Here's how the part is built. I have some questions about the finished solid (model axes, mm). A direction names the side the tool comes from. Coordinates: 2 decimals unless noted, no trailing zeros. Loops run counter-clockwise (first coordinate to the right, second up) from the corner with the lowest first, then second, coordinate; pieces in that order, holes last. Notation, with made-up numbers: M 15,13 L 19,13 A8 cw 19,18 Z; hole C 46,88 d2. An arc over 180 degrees is marked long. Use one line per item in the form item = value. Start each with the question number.
(1) Please list where these lines run through material, in increasing order: L1, parallel to X at y = -1.5, z = 1.5; L2, parallel to Z at x = 45.5, y = -1.3; L3, parallel to Z at x = 42, y = -1.
(2) Imagine slicing it at C-C, the plane z = 81. Please give me the cut outline in (x, y), and give its area (3 significant figures).
(3) On a 3-axis mill with a long thin cutter (end or side, diameter ignored), from which of +Z, -Z, +X, -X, +Y, -Y can I reach the whole of each face in a straight line? I mean faces 5 (the flat face through (14.527, -1.503, 40.216)), 6 (the flat face through (3, -3.048, 42)). Say none if no direction works.
(4) Thinking about a two-plate mould opening in Z: for faces 1 (the flat face through (-14.004, -1.503, 31.367)), 2 (the flat face through (3, 0, 42)), 3 (the flat face through (12.494, -1.503, 90.191)), 4 (the cylindrical face through (15.18, -1.5, 12.8)), which applies, +Z half, -Z half, draft (parallel to the pull), parting line (faces both ways), or undercut?
(5) Will this pin go through, and if not, where does the flat tip stop? P1, Ø1, axis at y = -0.5, z = 55.5, coming from the -X side.
(6) Imagine slicing it at B-B, the plane x = 6. Please give me the cut outline in (y, z).
(7) Imagine slicing it at A-A, the plane y = -1.85. State how many separate pieces and enclosed holes the cut face has, and give its area (3 significant figures).
```python
from build123d import *

# Parameters (mm, degrees)
F0_R     = 3.175
F1_DEPTH = 3.048


with BuildPart() as f1:
    # F0 (on Front) → F1 (new body)
    with BuildSketch(Plane.XZ):
        with BuildLine():
            Line((12.1285329959, 0), (3.175, 0))
            ThreePointArc((3.175, 0), (-2.2450640303, -2.2450640303), (0, 3.175))
            Line((0, 3.175), (0, 12.1285329959))
            ThreePointArc((0, 12.1285329959), (-8.8255371973, 8.3193272451), (-12.1074052539, -0.7155771445))
            ThreePointArc((-12.1074052539, -0.7155771445), (-7.858618829, -9.2381503956), (1.2349249899, -12.0654992811))
            ThreePointArc((1.2349249899, -12.0654992811), (9.002198096, -8.1278374782), (12.1285329959, 0))
        make_face()
        with BuildLine():
            ThreePointArc((0, 12.1285329959), (8.5761679272, 8.5761679272), (12.1285329959, 0))
            Line((12.1285329959, 0), (36.8473577956, 0))
            ThreePointArc((36.8473577956, 0), (39.3551513268, 5.6429323481), (45.2240996253, 7.5631301892))
            Line((45.2240996253, 7.5631301892), (20.3690705941, 10.1070859559))
            ThreePointArc((20.3690705941, 10.1070859559), (15.1229915635, 12.8646775774), (13.2422076318, 18.4850253022))
            Line((13.2422076318, 18.4850253022), (15.8473459627, 62.563383249))
            ThreePointArc((15.8473459627, 62.563383249), (10.8891421627, 51.9482811685), (0, 47.625))
            Line((0, 47.625), (0, 12.1285329959))
        make_face()
        with BuildLine():
            Line((36.8473577956, 0), (12.1285329959, 0))
            ThreePointArc((12.1285329959, 0), (9.002198096, -8.1278374782), (1.2349249899, -12.0654992811))
            Line((1.2349249899, -12.0654992811), (45.2240996253, -7.5631301892))
            ThreePointArc((45.2240996253, -7.5631301892), (39.3551513268, -5.6429323481), (36.8473577956, 0))
        make_face()
        with BuildLine():
            ThreePointArc((-12.1074052539, -0.7155771445), (-8.8255371973, 8.3193272451), (0, 12.1285329959))
            Line((0, 12.1285329959), (0, 47.625))
            ThreePointArc((0, 47.625), (-10.8891421627, 51.9482811685), (-15.8473459627, 62.563383249))
            Line((-15.8473459627, 62.563383249), (-12.1074052539, -0.7155771445))
        make_face()
        with BuildLine():
            ThreePointArc((45.2240996253, 7.5631301892), (39.3551513268, 5.6429323481), (36.8473577956, 0))
            ThreePointArc((36.8473577956, 0), (39.3551513268, -5.6429323481), (45.2240996253, -7.5631301892))
            ThreePointArc((45.2240996253, -7.5631301892), (50.0929323481, -5.0948486732), (52.0526422044, 0))
            ThreePointArc((52.0526422044, 0), (50.0929323481, 5.0948486732), (45.2240996253, 7.5631301892))
        make_face()
        with BuildLine():
            ThreePointArc((47.625, 0), (44.45, -3.175), (41.275, 0))
            ThreePointArc((41.275, 0), (44.45, 3.175), (47.625, 0))
        make_face(mode=Mode.SUBTRACT)
        with BuildLine():
            ThreePointArc((-15.8473459627, 62.563383249), (-10.8891421627, 51.9482811685), (0, 47.625))
            Line((0, 47.625), (0, 60.325))
            ThreePointArc((0, 60.325), (-3.175, 63.5), (0, 66.675))
            Line((0, 66.675), (0, 79.375))
            ThreePointArc((0, 79.375), (-10.4661659349, 75.4362890222), (-15.7388575186, 65.5746057477))
            ThreePointArc((-15.7388575186, 65.5746057477), (-15.8647069883, 64.071574295), (-15.8473459627, 62.563383249))
        make_face()
        with BuildLine():
            Line((0, 60.325), (0, 47.625))
            ThreePointArc((0, 47.625), (10.8891421627, 51.9482811685), (15.8473459627, 62.563383249))
            ThreePointArc((15.8473459627, 62.563383249), (15.8680849846, 63.0314875444), (15.875, 63.5))
            ThreePointArc((15.875, 63.5), (15.8409278154, 64.5395340042), (15.7388575186, 65.5746057477))
            ThreePointArc((15.7388575186, 65.5746057477), (10.4661659349, 75.4362890222), (0, 79.375))
            Line((0, 79.375), (0, 66.675))
            ThreePointArc((0, 66.675), (2.2450640303, 65.7450640303), (3.175, 63.5))
            ThreePointArc((3.175, 63.5), (2.2450640303, 61.2549359697), (0, 60.325))
        make_face()
        with BuildLine():
            Line((-9.1570523114, 115.5070300106), (-15.7388575186, 65.5746057477))
            ThreePointArc((-15.7388575186, 65.5746057477), (-10.4661659349, 75.4362890222), (0, 79.375))
            Line((0, 79.375), (0, 105.0637383927))
            ThreePointArc((0, 105.0637383927), (-6.9446732617, 108.2106616314), (-9.1570523114, 115.5070300106))
        make_face()
        with Locations((-3.6322516389, 98.6820235848)):
            Circle(F0_R, mode=Mode.SUBTRACT)
        with BuildLine():
            Line((0, 105.0637383927), (0, 79.375))
            ThreePointArc((0, 79.375), (10.4661659349, 75.4362890222), (15.7388575186, 65.5746057477))
            Line((15.7388575186, 65.5746057477), (9.1570523114, 115.5070300106))
            ThreePointArc((9.1570523114, 115.5070300106), (9.2164380099, 114.9048131032), (9.2362616073, 114.3))
            ThreePointArc((9.2362616073, 114.3), (6.5310232154, 107.7689767846), (0, 105.0637383927))
        make_face()
        with BuildLine():
            ThreePointArc((9.1570523114, 115.5070300106), (0, 123.5362616073), (-9.1570523114, 115.5070300106))
            ThreePointArc((-9.1570523114, 115.5070300106), (-6.9446732617, 108.2106616314), (0, 105.0637383927))
            ThreePointArc((0, 105.0637383927), (6.5310232154, 107.7689767846), (9.2362616073, 114.3))
            ThreePointArc((9.2362616073, 114.3), (9.2164380099, 114.9048131032), (9.1570523114, 115.5070300106))
        make_face()
        with BuildLine():
            ThreePointArc((3.175, 114.3), (2.2450640303, 112.0549359697), (0, 111.125))
            ThreePointArc((0, 111.125), (-2.2450640303, 116.5450640303), (3.175, 114.3))
        make_face(mode=Mode.SUBTRACT)
        with BuildLine():
            ThreePointArc((0, 3.175), (2.2450640303, 2.2450640303), (3.175, 0))
            Line((3.175, 0), (12.1285329959, 0))
            ThreePointArc((12.1285329959, 0), (8.5761679272, 8.5761679272), (0, 12.1285329959))
            Line((0, 12.1285329959), (0, 3.175))
        make_face()
    extrude(amount=F1_DEPTH)


solid = f1.part
```
Answer:
q1.L1 = -12.24 to -2.8, 2.8 to 41.65, 47.25 to 51.9
q1.L2 = -7.53 to -3, 3 to 7.53
q1.L3 = -7.89 to -2.02, 2.02 to 7.89
q2.outline = M -13.71,-3.05 L 13.71,-3.05 L 13.71,0 L -13.71,0 Z
q2.area = 83.5 mm²
q3.face_5 = +X, +Y, -Y
q3.face_6 = +Z, -Z, +X, -X, -Y
q4.face_1 = -Z half
q4.face_2 = draft
q4.face_3 = +Z half
q4.face_4 = undercut
q5.P1 = -15.46
q6.outline = M -3.05,-11.58 L 0,-11.58 L 0,121.32 L -3.05,121.32 Z
q7.separate_pieces = 1
q7.enclosed_holes = 5
q7.area = 4,000 mm²
